from build123d import *

# Parameters (mm, degrees)
F0_W         = 95.0192604214
F0_H         = 18.9093053341
F1_DEPTH     = 1.6002
F2_R         = 1.4351
F3_DEPTH     = 25.4
F4_R         = 1.397
F5_DEPTH     = 2.54
F6_W         = 48.927821219
F6_H         = 30.7276230305
F7_DEPTH     = 3.6195
F8_T1_DEPTH  = 30.6197
F8_T6_DEPTH  = 56.1276230305
F8_T12_DEPTH = 56.1276230305
F8_T18_DEPTH = 56.1276230305
F8_T25_DEPTH = 56.1276230305
F8_T31_DEPTH = 56.1276230305
F8_T37_DEPTH = 56.1276230305
F8_T43_DEPTH = 56.1276230305
F8_T49_DEPTH = 56.1276230305
F8_T56_DEPTH = 56.1276230305
F8_T62_DEPTH = 56.1276230305
F9_T1_DEPTH  = 37.4142992276
F10_R        = 12.7
F12_R        = 33.1286185238
F13_DEPTH    = 102.87
F14_W        = 25.4
F14_H        = 4.064
F15_DEPTH    = 38.1


# Not quite as in the source:
# - a fillet or chamfer that OpenCascade refuses, or shapes differently, is made with other operations: its cross-section is extruded or revolved along the edge and cut away or added


with BuildPart() as f1:
    # F0 (on Top) → F1 (new body)
    with BuildSketch(Plane.XY):
        Polygon((-24.4639106095, -15.3638115153), (24.4639106095, -15.3638115153), (24.4639106095, -9.454652667), (24.4639106095, 9.454652667), (24.4639106095, 15.3638115153), (-24.4639106095, 15.3638115153), (-24.4639106095, 9.454652667), (-24.4639106095, -9.454652667), align=None)
        with Locations((71.9735408202, 0)):
            Rectangle(F0_W, F0_H)
        with Locations((-71.9735408202, 0)):
            Rectangle(F0_W, F0_H)
    extrude(amount=F1_DEPTH)

    # F2 (on face) → F3 (cut)
    with BuildSketch(Plane.XY.offset(1.6002)):
        with Locations((106.7831710309, 0)):
            Circle(F2_R)
        with Locations((94.0831710309, 0)):
            Circle(F2_R)
        with Locations((81.3831710309, 0)):
            Circle(F2_R)
        with Locations((68.6831710309, 0)):
            Circle(F2_R)
        with Locations((55.9831710309, 0)):
            Circle(F2_R)
        with Locations((43.2831710309, 0)):
            Circle(F2_R)
    extrude(amount=-F3_DEPTH, mode=Mode.SUBTRACT)

    # F4 (on face) → F5 (join)
    with BuildSketch(Plane.XY.offset(1.6002)):
        with Locations((-106.7719441229, 0)):
            Circle(F4_R)
        with Locations((-94.0719441229, 0)):
            Circle(F4_R)
        with Locations((-81.3719441229, 0)):
            Circle(F4_R)
        with Locations((-68.6719441229, 0)):
            Circle(F4_R)
        with Locations((-55.9719441229, 0)):
            Circle(F4_R)
        with Locations((-43.2719441229, 0)):
            Circle(F4_R)
    extrude(amount=F5_DEPTH)

    # F6 (on face) → F7 (join)
    with BuildSketch(Plane.XY.offset(1.6002)):
        Rectangle(F6_W, F6_H)
    extrude(amount=F7_DEPTH)

    # F8: fillet of radius 5.08 on 6 edges, made by hand

    # F8_s2 → F8_t1 (cut)
    with BuildSketch(Plane.XY.offset(-12.7)):
        with BuildLine():
            ThreePointArc((-19.3839106095, 15.3638115153), (-22.9760130579, 13.8759139637), (-24.4639106095, 10.2838115153))
            Line((-24.4639106095, 10.2838115153), (-24.4639106095, 15.3638115153))
            Line((-24.4639106095, 15.3638115153), (-19.3839106095, 15.3638115153))
        make_face()
        with BuildLine():
            ThreePointArc((-19.3839106095, -15.3638115153), (-22.9760130579, -13.8759139637), (-24.4639106095, -10.2838115153))
            Line((-24.4639106095, -10.2838115153), (-24.4639106095, -15.3638115153))
            Line((-24.4639106095, -15.3638115153), (-19.3839106095, -15.3638115153))
        make_face()
        with BuildLine():
            ThreePointArc((19.3839106095, -15.3638115153), (22.9760130579, -13.8759139637), (24.4639106095, -10.2838115153))
            Line((24.4639106095, -10.2838115153), (24.4639106095, -15.3638115153))
            Line((24.4639106095, -15.3638115153), (19.3839106095, -15.3638115153))
        make_face()
        with BuildLine():
            ThreePointArc((19.3839106095, 15.3638115153), (22.9760130579, 13.8759139637), (24.4639106095, 10.2838115153))
            Line((24.4639106095, 10.2838115153), (24.4639106095, 15.3638115153))
            Line((24.4639106095, 15.3638115153), (19.3839106095, 15.3638115153))
        make_face()
    extrude(amount=F8_T1_DEPTH, mode=Mode.SUBTRACT)


with BuildPart() as f8_tool4:
    # F8_s5 → F8_t6 (new body)
    with BuildSketch(Plane.XZ.offset(28.0638115153)):
        with BuildLine():
            ThreePointArc((24.4639106095, 0.1397), (22.9760130579, 3.7318024484), (19.3839106095, 5.2197))
            Line((19.3839106095, 5.2197), (24.4639106095, 5.2197))
            Line((24.4639106095, 5.2197), (24.4639106095, 0.1397))
        make_face()
    extrude(amount=-F8_T6_DEPTH)

    split(bisect_by=Plane.XY.offset(1.6002), keep=Keep.BOTTOM)

    split(bisect_by=Plane.XZ.offset(9.454652667), keep=Keep.TOP)


with BuildPart() as f1_1:
    add(f1.part)

    # F8_t3: cut F8_tool4
    add(f8_tool4.part, mode=Mode.SUBTRACT)


with BuildPart() as f8_tool10:
    # F8_s11 → F8_t12 (new body)
    with BuildSketch(Plane.XZ.offset(28.0638115153)):
        with BuildLine():
            ThreePointArc((24.4639106095, 0.1397), (22.9760130579, 3.7318024484), (19.3839106095, 5.2197))
            Line((19.3839106095, 5.2197), (24.4639106095, 5.2197))
            Line((24.4639106095, 5.2197), (24.4639106095, 0.1397))
        make_face()
    extrude(amount=-F8_T12_DEPTH)

    split(bisect_by=Plane.XY.offset(1.6002), keep=Keep.TOP)

    split(bisect_by=Plane.XZ.offset(9.454652667), keep=Keep.TOP)


with BuildPart() as f1_2:
    add(f1_1.part)

    # F8_t9: cut F8_tool10
    add(f8_tool10.part, mode=Mode.SUBTRACT)


with BuildPart() as f8_tool16:
    # F8_s17 → F8_t18 (new body)
    with BuildSketch(Plane.XZ.offset(28.0638115153)):
        with BuildLine():
            ThreePointArc((24.4639106095, 0.1397), (22.9760130579, 3.7318024484), (19.3839106095, 5.2197))
            Line((19.3839106095, 5.2197), (24.4639106095, 5.2197))
            Line((24.4639106095, 5.2197), (24.4639106095, 0.1397))
        make_face()
    extrude(amount=-F8_T18_DEPTH)

    split(bisect_by=Plane.XY.offset(1.6002), keep=Keep.TOP)

    split(bisect_by=Plane.XZ.offset(-9.454652667), keep=Keep.TOP)

    split(bisect_by=Plane.XZ.offset(9.454652667), keep=Keep.BOTTOM)


with BuildPart() as f1_3:
    add(f1_2.part)

    # F8_t15: cut F8_tool16
    add(f8_tool16.part, mode=Mode.SUBTRACT)


with BuildPart() as f8_tool23:
    # F8_s24 → F8_t25 (new body)
    with BuildSketch(Plane.XZ.offset(28.0638115153)):
        with BuildLine():
            ThreePointArc((24.4639106095, 0.1397), (22.9760130579, 3.7318024484), (19.3839106095, 5.2197))
            Line((19.3839106095, 5.2197), (24.4639106095, 5.2197))
            Line((24.4639106095, 5.2197), (24.4639106095, 0.1397))
        make_face()
    extrude(amount=-F8_T25_DEPTH)

    split(bisect_by=Plane.XY.offset(1.6002), keep=Keep.BOTTOM)

    split(bisect_by=Plane.XZ.offset(-9.454652667), keep=Keep.BOTTOM)


with BuildPart() as f1_4:
    add(f1_3.part)

    # F8_t22: cut F8_tool23
    add(f8_tool23.part, mode=Mode.SUBTRACT)


with BuildPart() as f8_tool29:
    # F8_s30 → F8_t31 (new body)
    with BuildSketch(Plane.XZ.offset(28.0638115153)):
        with BuildLine():
            ThreePointArc((24.4639106095, 0.1397), (22.9760130579, 3.7318024484), (19.3839106095, 5.2197))
            Line((19.3839106095, 5.2197), (24.4639106095, 5.2197))
            Line((24.4639106095, 5.2197), (24.4639106095, 0.1397))
        make_face()
    extrude(amount=-F8_T31_DEPTH)

    split(bisect_by=Plane.XY.offset(1.6002), keep=Keep.TOP)

    split(bisect_by=Plane.XZ.offset(-9.454652667), keep=Keep.BOTTOM)


with BuildPart() as f1_5:
    add(f1_4.part)

    # F8_t28: cut F8_tool29
    add(f8_tool29.part, mode=Mode.SUBTRACT)


with BuildPart() as f8_tool35:
    # F8_s36 → F8_t37 (new body)
    with BuildSketch(Plane.XZ.offset(-28.0638115153)):
        with BuildLine():
            ThreePointArc((-19.3839106095, 5.2197), (-22.9760130579, 3.7318024484), (-24.4639106095, 0.1397))
            Line((-24.4639106095, 0.1397), (-24.4639106095, 5.2197))
            Line((-24.4639106095, 5.2197), (-19.3839106095, 5.2197))
        make_face()
    extrude(amount=F8_T37_DEPTH)

    split(bisect_by=Plane.XZ.offset(-9.454652667), keep=Keep.BOTTOM)

    split(bisect_by=Plane.XY.offset(1.6002), keep=Keep.TOP)


with BuildPart() as f1_6:
    add(f1_5.part)

    # F8_t34: cut F8_tool35
    add(f8_tool35.part, mode=Mode.SUBTRACT)


with BuildPart() as f8_tool41:
    # F8_s42 → F8_t43 (new body)
    with BuildSketch(Plane.XZ.offset(-28.0638115153)):
        with BuildLine():
            ThreePointArc((-19.3839106095, 5.2197), (-22.9760130579, 3.7318024484), (-24.4639106095, 0.1397))
            Line((-24.4639106095, 0.1397), (-24.4639106095, 5.2197))
            Line((-24.4639106095, 5.2197), (-19.3839106095, 5.2197))
        make_face()
    extrude(amount=F8_T43_DEPTH)

    split(bisect_by=Plane.XZ.offset(-9.454652667), keep=Keep.BOTTOM)

    split(bisect_by=Plane.XY.offset(1.6002), keep=Keep.BOTTOM)


with BuildPart() as f1_7:
    add(f1_6.part)

    # F8_t40: cut F8_tool41
    add(f8_tool41.part, mode=Mode.SUBTRACT)


with BuildPart() as f8_tool47:
    # F8_s48 → F8_t49 (new body)
    with BuildSketch(Plane.XZ.offset(-28.0638115153)):
        with BuildLine():
            ThreePointArc((-19.3839106095, 5.2197), (-22.9760130579, 3.7318024484), (-24.4639106095, 0.1397))
            Line((-24.4639106095, 0.1397), (-24.4639106095, 5.2197))
            Line((-24.4639106095, 5.2197), (-19.3839106095, 5.2197))
        make_face()
    extrude(amount=F8_T49_DEPTH)

    split(bisect_by=Plane.XZ.offset(-9.454652667), keep=Keep.TOP)

    split(bisect_by=Plane.XY.offset(1.6002), keep=Keep.TOP)

    split(bisect_by=Plane.XZ.offset(9.454652667), keep=Keep.BOTTOM)


with BuildPart() as f1_8:
    add(f1_7.part)

    # F8_t46: cut F8_tool47
    add(f8_tool47.part, mode=Mode.SUBTRACT)


with BuildPart() as f8_tool54:
    # F8_s55 → F8_t56 (new body)
    with BuildSketch(Plane.XZ.offset(-28.0638115153)):
        with BuildLine():
            ThreePointArc((-19.3839106095, 5.2197), (-22.9760130579, 3.7318024484), (-24.4639106095, 0.1397))
            Line((-24.4639106095, 0.1397), (-24.4639106095, 5.2197))
            Line((-24.4639106095, 5.2197), (-19.3839106095, 5.2197))
        make_face()
    extrude(amount=F8_T56_DEPTH)

    split(bisect_by=Plane.XY.offset(1.6002), keep=Keep.TOP)

    split(bisect_by=Plane.XZ.offset(9.454652667), keep=Keep.TOP)


with BuildPart() as f1_9:
    add(f1_8.part)

    # F8_t53: cut F8_tool54
    add(f8_tool54.part, mode=Mode.SUBTRACT)


with BuildPart() as f8_tool60:
    # F8_s61 → F8_t62 (new body)
    with BuildSketch(Plane.XZ.offset(-28.0638115153)):
        with BuildLine():
            ThreePointArc((-19.3839106095, 5.2197), (-22.9760130579, 3.7318024484), (-24.4639106095, 0.1397))
            Line((-24.4639106095, 0.1397), (-24.4639106095, 5.2197))
            Line((-24.4639106095, 5.2197), (-19.3839106095, 5.2197))
        make_face()
    extrude(amount=F8_T62_DEPTH)

    split(bisect_by=Plane.XY.offset(1.6002), keep=Keep.BOTTOM)

    split(bisect_by=Plane.XZ.offset(9.454652667), keep=Keep.TOP)


with BuildPart() as f1_10:
    add(f1_9.part)

    # F8_t59: cut F8_tool60
    add(f8_tool60.part, mode=Mode.SUBTRACT)

    # F9: fillet of radius 5.08 on 2 edges, made by hand

    # F9_s2 → F9_t1 (cut)
    with BuildSketch(Plane.XZ.offset(-18.7071496138)):
        with BuildLine():
            ThreePointArc((115.7821722522, 1.6002), (117.7982347512, 1.1830201767), (119.4831710309, 0))
            Line((119.4831710309, 0), (119.4831710309, 1.6002))
            Line((119.4831710309, 1.6002), (115.7821722522, 1.6002))
        make_face()
        with BuildLine():
            ThreePointArc((-119.4831710309, 0), (-117.7982347512, 1.1830201767), (-115.7821722522, 1.6002))
            Line((-115.7821722522, 1.6002), (-119.4831710309, 1.6002))
            Line((-119.4831710309, 1.6002), (-119.4831710309, 0))
        make_face()
    extrude(amount=F9_T1_DEPTH, mode=Mode.SUBTRACT)

    # F10
    f10_edges = [f1_10.edges().sort_by_distance(p)[0] for p in [
        (24.249436, 0, 1.6002),
        (-24.249436, 0, 1.6002),
    ]]
    fillet(f10_edges, radius=F10_R)

    # F12 (on offset) → F13 (cut)
    with BuildSketch(Plane.YZ.offset(-19.3802)):
        Circle(F12_R)
    extrude(amount=-F13_DEPTH, mode=Mode.SUBTRACT)

    # F14 (on offset) → F15 (cut)
    with BuildSketch(Plane.YZ.offset(-19.3802)):
        with Locations((0, 4.0005)):
            Rectangle(F14_W, F14_H)
    extrude(amount=F15_DEPTH, mode=Mode.SUBTRACT)


solid = f1_10.part
Part model, mm, in its own coordinate system. A direction names the side the tool comes from. Coordinates: 2 decimals unless noted, no trailing zeros. Order: outer loops, then holes, each group sorted by start corner. A loop starts at its lowest first (then second) coordinate and runs counter-clockwise, first axis right, second up.
(1) Probe L1, parallel to Y at x = 11.5, z = 2.25; L2, parallel to Z at x = 89, y = 0; L3, parallel to Y at x = 87.5, z = 0.4. List the from-to ranges inside material, lowest first.
Check sheet entries:
L1: y = -15.36 to -12.7, 12.7 to 15.36
L2: z = 0 to 1.6
L3: y = -9.45 to 9.45
(2) Slice it at A-A, the plane y = 0. State how many separate pieces and enclosed holes the cut face has, and give its area (3 significant figures).
Check sheet entries:
separate pieces: 7
enclosed holes: 0
area: 226 mm2
(3) Slice it at B-B, the plane y = -7. Write the cut outline in (x, z).
Check sheet entries:
outline: (-19.38, 0) - (119.48, 0) arc R5.08 ccw to (115.78, 1.6) - (30.14, 1.6) arc R12.7 cw to (22.46, 4.19) arc R5.08 ccw to (19.38, 5.22) - (18.72, 5.22) - (18.72, 1.97) - (-19.38, 1.97) - close
(4) Pull direction X, two halves, no side cores. Call faces 1 (the face through (108.152, 0.431, 0.811)), 2 (the face through (95.452, 0.431, 0.811)), 3 (the face through (18.72, 0, 4)), 4 (the face through (-1, 12.7, 4)): pulls with the +X half, pulls with the -X half, needs draft (parallel to the pull), parting line crosses it, or undercut.
Check sheet entries:
face 1: undercut
face 2: undercut
face 3: pulls with the -X half
face 4: needs draft
(5) Tool access for faces 5 (the face through (-19.38, 0, 1)), 6 (the face through (-1, -12.7, 4)): list every direction of +Z, -Z, +X, -X, +Y, -Y with a clear straight run to the whole face (end or side of a thin tool).
Check sheet entries:
face 5: +Z, -Z, -X, +Y, -Y
face 6: +Z, -X
(6) Slice it at C-C, the plane x = 76.5. Write the cut outline in (y, z), and give its area (3 significant figures).
Check sheet entries:
outline: (-9.45, 0) - (9.45, 0) - (9.45, 1.6) - (-9.45, 1.6) - close
area: 30.3 mm2
(7) Pin check, flat tips, straight feed: pin 1 Ø1.7 at (x, y) = (68.68, 0) entering from +Z; pin 2 Ø9.5 at (x, y) = (70, -1.5) entering from +Z; pin 3 Ø12.5 at (x, y) = (6.5, -3.5) entering from +Z. Stop position of each tip, or through.
Check sheet entries:
pin 1: passes through
pin 2: stops at z = 1.6
pin 3: stops at z = 1.97
